Check sheet for the modelled part. Datum: model origin and axes. Units: mm. A direction names the side the tool comes from. Round coordinates to 2 decimals unless told otherwise and drop trailing zeros. Order: outer loops, then holes, each group sorted by start corner. A loop starts at its lowest first (then second) coordinate and runs counter-clockwise, first axis right, second up.
from build123d import *

# Parameters (mm, degrees)
F0_W     = 150
F0_H     = 50
F0_W_2   = 50
F0_W_3   = 100
F1_DEPTH = 25


with BuildPart() as f1:
    # F0 (on Top) → F1 (new body)
    with BuildSketch(Plane.XY):
        with Locations((26.636132, 125)):
            Rectangle(F0_W, F0_H)
        with Locations((-73.363868, 125)):
            Rectangle(F0_W_2, F0_H)
        with Locations((-73.363868, 75)):
            Rectangle(F0_W_2, F0_H)
        with Locations((1.636132, 25)):
            Rectangle(F0_W_3, F0_H)
        with Locations((-73.363868, 25)):
            Rectangle(F0_W_2, F0_H)
        with Locations((76.636132, 25)):
            Rectangle(F0_W_2, F0_H)
        with Locations((76.636132, -25)):
            Rectangle(F0_W_2, F0_H)
        with Locations((76.636132, -75)):
            Rectangle(F0_W_2, F0_H)
        with Locations((-23.363868, -75)):
            Rectangle(F0_W, F0_H)
    extrude(amount=F1_DEPTH)


solid = f1.part
1) Sectioned sample at A-A on x = 80.5. Record the cut outline in (y, z).
2) Scan lines: line 1 (Y direction, x = -6, z = 12); line 2 (Y direction, x = 78.5, z = 23); line 3 (Y direction, x = -67.5, z = 12.5). Record each from-to range of solid material in increasing order.
3) Draft check along Y on faces 1 (the face through (-48.364, 75, 12)), 2 (the face through (3, 150, 12)), 3 (the face through (101.636, 125, 12)), 4 (the face through (26, 100, 12)). Enter one of: pulls with the +Y half, pulls with the -Y half, needs draft (parallel to the pull), parting line crosses it, or undercut.
4) Sectioned sample at C-C on z = 3.25. Record the cut outline in (x, y), and give its area (3 significant figures).
5) Gauge pin test, flat ends, axial feed: pin 1 (7.5 mm diameter, centred on y = 80, z = 6.5, fed in from +X); pin 2 (4 mm diameter, centred on x = -51, y = 45, fed in from -Z). Record the tip position at first contact, or that the pin passes through.
6) Sectioned sample at B-B on x = 12. Record the cut outline in (y, z).
7) Sectioned sample at D-D on y = -6. Record the cut outline in (x, z).
8) Set-up check for faces 5 (the face through (-24, -50, 12)), 6 (the face through (28, 50, 12)), 7 (the face through (0, 27, 0)): record each of +Z, -Z, +X, -X, +Y, -Y from which the full face is reachable in a straight line by a thin tool's end or side.
Values found:
1. outline: (-100, 0) - (50, 0) - (50, 25) - (-100, 25) - close; (100, 0) - (150, 0) - (150, 25) - (100, 25) - close
2. line 1: y = -100 to -50, 0 to 50, 100 to 150
2. line 2: y = -100 to 50, 100 to 150
2. line 3: y = -100 to -50, 0 to 150
3. face 1: undercut
3. face 2: pulls with the +Y half
3. face 3: needs draft
3. face 4: undercut
4. outline: (-98.36, -100) - (101.64, -100) - (101.64, 50) - (-48.36, 50) - (-48.36, 100) - (101.64, 100) - (101.64, 150) - (-98.36, 150) - (-98.36, 0) - (51.64, 0) - (51.64, -50) - (-98.36, -50) - close
4. area: 35,000 mm2
5. pin 1: stops at x = -48.36
5. pin 2: stops at z = 0
6. outline: (-100, 0) - (-50, 0) - (-50, 25) - (-100, 25) - close; (0, 0) - (50, 0) - (50, 25) - (0, 25) - close; (100, 0) - (150, 0) - (150, 25) - (100, 25) - close
7. outline: (51.64, 0) - (101.64, 0) - (101.64, 25) - (51.64, 25) - close
8. face 5: +Z, -Z, -X
8. face 6: +Z, -Z, +X
8. face 7: -Z, +X, -X, +Y, -Y
